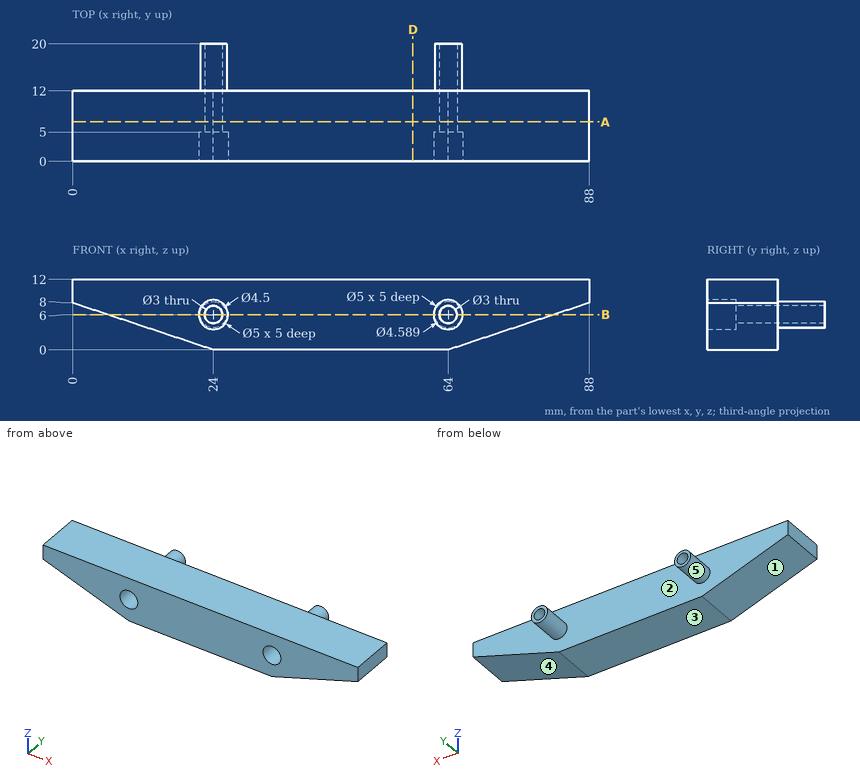
Study the drawing (mm; zero at the part's minimum x, y, z) and answer. A direction names the side the tool comes from. Round coordinates to 2 decimals unless told otherwise and drop trailing zeros. Write each loop counter-clockwise with the first axis right and the second up, starting at its lowest first coordinate (ties: lowest second). Pieces come first, ordered by that corner, then holes.
Q1. Find section A-A on y = 6.75. Determine the outline of the cut face in (x, z), and give its area (3 significant figures).
Values:
outline: (0, 8) - (24, 0) - (64, 0) - (88, 8) - (88, 12) - (0, 12) - close; hole circle Ø3 at (24, 6); hole circle Ø3 at (64, 6)
area: 850 mm2
Q2. Find section B-B on z = 6. State how many separate pieces and enclosed holes the cut face has, and give its area (3 significant figures).
Values:
separate pieces: 3
enclosed holes: 0
area: 845 mm2
Q3. The mould has two halves that part along X. Classify the marked faces 1, 2 and 3: released by +X, released by -X, zero draft, split by the parting line, or undercut.
Values:
face 1: released by -X
face 2: undercut
face 3: zero draft
Q4. Straight lines are drawn through the part: line 1 (Z direction, x = 64, y = 11.5); line 2 (Y direction, x = 36, z = 7); line 3 (Z direction, x = 66.5, y = 7.25). For each, find the intervals that lie inside material, in ascending order.
Values:
line 1: z = 0 to 4.5, 7.5 to 12
line 2: y = 0 to 12
line 3: z = 0.83 to 12
Q5. A tool of negligible diameter and unlimited length cuts with its end or side. For the marked faces 4 and 5, from which of +Z, -Z, +X, -X, +Y, -Y can it reach the whole face along a straight path? Write none if from no direction.
Values:
face 4: -Z, +X, +Y, -Y
face 5: +Y
Q6. Flat-ended cylindrical pins translate along their axes: P1, Ø1.5, axis at x = 24, y = 15.5, coming from the -Z side; P2, Ø6, axis at x = 76, z = 1.5, coming from the +Y side; P3, Ø2.5, axis at x = 23.5, z = 6, coming from the -Y side; P4, Ø1.8, axis at x = 24, z = 6, coming from the +Y side. Find the tip coordinate at first contact, or state that the pin passes through.
Values:
P1: stops at z = 3.75
P2: stops at y = 12
P3: stops at y = 5
P4: passes through
Q7. Find section D-D on x = 58. Determine the outline of the cut face in (y, z).
Values:
outline: (0, 0) - (12, 0) - (12, 12) - (0, 12) - close
